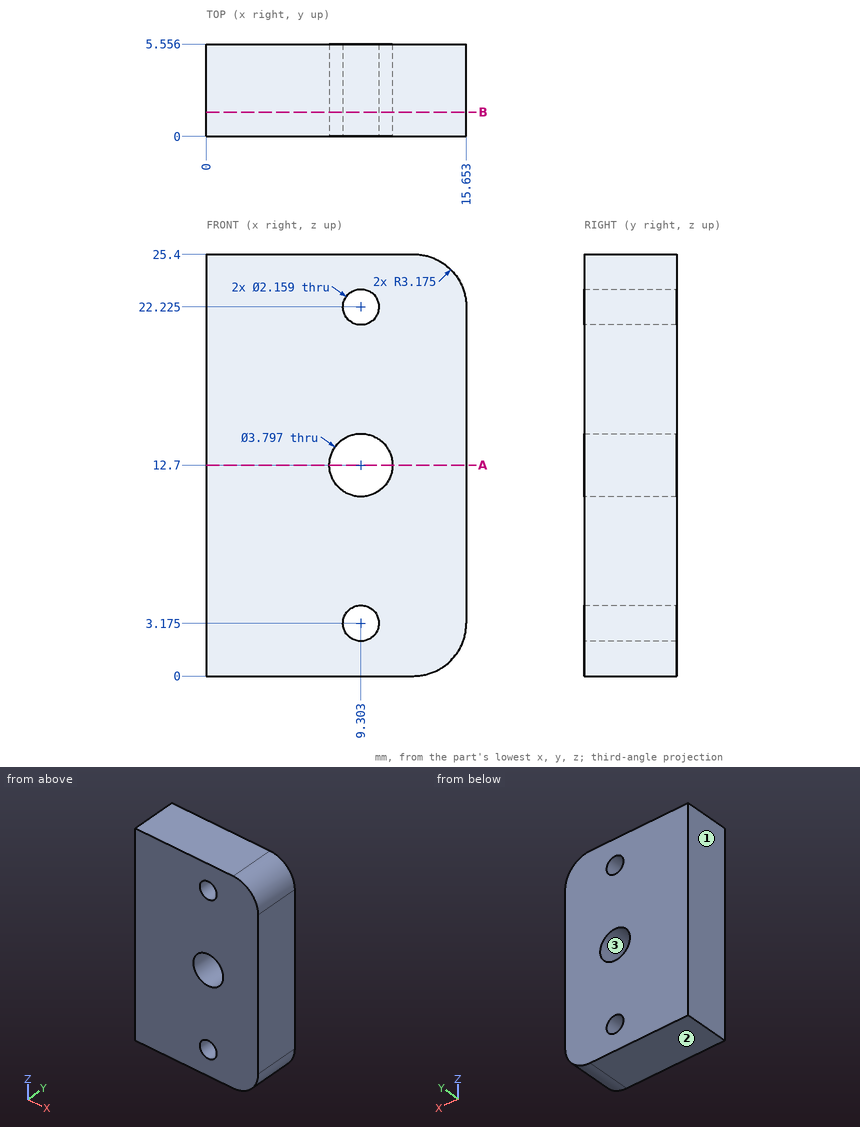
Geometry: see drawing. Coordinates: mm, zero at the bounding-box minimum. Coordinates: 2 decimals unless noted, no trailing zeros. Loops run counter-clockwise (first coordinate to the right, second up) from the corner with the lowest first, then second, coordinate; pieces in that order, holes last.
(1) Material intervals for probe 1 along X at (y, z) = (4.1, 12.7); probe 2 along Z at (x, y) = (10.25, 4.15) (1 decimal); probe 3 along Z at (x, y) = (8.75, 2.4), sorted ascending.
(2) Section A-A on z = 12.7. Return the cut outline in (x, y).
(3) Section B-B on y = 1.45. Count the separate pieces of the cut face and the enclosed holes in it, then the cut area to 3 significant figures.
(4) Pull-direction query (Z, two-part tool) for the marked faces 1, 2 and 3; classes: released by +Z, released by -Z, zero draft, split by the parting line, or undercut.
(5) First-contact query: pin 1 Ø6 at (x, z) = (7, 11) entering from -Y; pin 2 Ø1.9 at (x, z) = (9.3, 22.22) entering from +Y. Flat tips, straight axial feed; report the tip coordinate or a pass-through.
Data:
1. probe 1: x = 0 to 7.4, 11.2 to 15.65
1. probe 2: z = 0 to 2.7, 3.7 to 11.1, 14.3 to 21.7, 22.7 to 25.4
1. probe 3: z = 0 to 2.25, 4.1 to 10.88, 14.52 to 21.3, 23.15 to 25.4
2. outline: (0, 0) - (7.4, 0) - (7.4, 5.56) - (0, 5.56) - close; (11.2, 0) - (15.65, 0) - (15.65, 5.56) - (11.2, 5.56) - close
3. separate pieces: 1
3. enclosed holes: 3
3. area: 375 mm2
4. face 1: zero draft
4. face 2: released by -Z
4. face 3: undercut
5. pin 1: stops at y = 0
5. pin 2: passes through
